from build123d import *

# Parameters (mm, degrees)
BOSS_EXTRUDE1_DEPTH = 5
SKETCH1_3_R         = 10
BOSS_EXTRUDE2_DEPTH = 2.5


with BuildPart() as part:
    # Sketch1 → Boss-Extrude1 (new, symmetric)
    with BuildSketch(Plane.XY):
        with BuildLine():
            Line((33, 85), (-32, 85))
            ThreePointArc((-32, 85), (-48.980483062, 75.567080721), (-49.943413521, 56.166319497))
            Line((-49.943413521, 56.166319497), (-17.943413521, -8.833680503))
            ThreePointArc((-17.943413521, -8.833680503), (0, -20), (17.943413521, -8.833680503))
            Line((17.943413521, -8.833680503), (50.833146609, 55.945780983))
            ThreePointArc((50.833146609, 55.945780983), (50.045298184, 75.46220865), (33, 85))
        make_face()
        with BuildLine():
            ThreePointArc((13.317368267, 6.90273152), (0, -15), (-13.317368267, 6.90273152))
            ThreePointArc((-13.317368267, 6.90273152), (-13.036984521, 33.958715313), (-34.650701601, 50.236064853))
            ThreePointArc((-34.650701601, 50.236064853), (-45.218522192, 72.090181314), (-21.166666667, 75.374916332))
            ThreePointArc((-21.166666667, 75.374916332), (0.5, 66.124748995), (22.166666667, 75.374916332))
            ThreePointArc((22.166666667, 75.374916332), (46.692872743, 71.124151864), (33.511719921, 50.008731117))
            ThreePointArc((33.511719921, 50.008731117), (12.785531325, 33.43522428), (13.317368267, 6.90273152))
        make_face(mode=Mode.SUBTRACT)
    extrude(amount=BOSS_EXTRUDE1_DEPTH, both=True)

    # Sketch1_3 → Boss-Extrude2 (add, symmetric)
    with BuildSketch(Plane.XY):
        with BuildLine():
            Line((-32, 85), (33, 85))
            ThreePointArc((33, 85), (50.045298184, 75.46220865), (50.833146609, 55.945780983))
            Line((50.833146609, 55.945780983), (17.943413521, -8.833680503))
            ThreePointArc((17.943413521, -8.833680503), (0, -20), (-17.943413521, -8.833680503))
            Line((-17.943413521, -8.833680503), (-49.943413521, 56.166319497))
            ThreePointArc((-49.943413521, 56.166319497), (-48.980483062, 75.567080721), (-32, 85))
        make_face()
        with Locations((-32, 65)):
            Circle(SKETCH1_3_R, mode=Mode.SUBTRACT)
        with Locations((33, 65)):
            Circle(SKETCH1_3_R, mode=Mode.SUBTRACT)
        Circle(SKETCH1_3_R, mode=Mode.SUBTRACT)
    extrude(amount=BOSS_EXTRUDE2_DEPTH, both=True)


solid = part.part
Check sheet for the modelled part. Datum: model origin and axes. Units: mm. A direction names the side the tool comes from. Round coordinates to 2 decimals unless told otherwise and drop trailing zeros. Write each loop counter-clockwise with the first axis right and the second up, starting at its lowest first coordinate (ties: lowest second). Pieces come first, ordered by that corner, then holes. Notation, with made-up numbers: (60, 78.25) -> (93, 78.25) arc R16 ccw to (93, 104.25) -> close; hole circle Ø11 at (72, -33). An arc over 180 degrees is marked (long way). Answer as CSV lines item,"result". Start each with the question number.
1) Material ranges on line 1 (Z direction, x = -9.5, y = 43); line 2 (Y direction, x = 0, z = 3.3); line 3 (Y direction, x = -32, z = -3.3), recorded low to high. Write a range as from..to.
2) Tool access check on faces 5 (the cylindrical face through (0, -15, 4)), 6 (the flat face through (-15, 37, -5)), 7 (the cylindrical face through (-12.87, 33.61, -3.73)). Record the directions out of +Z, -Z, +X, -X, +Y, -Y that give a thin tool (end or side, any length) a straight path to the whole face; none if there is none.
3) Section check B-B on y = 0. Enter the section's corners in (x, z).
4) Go/stop test with flat-tipped pins: P1, Ø24, axis at x = 0, y = 0, coming from the +Z side; P2, Ø1.5, axis at x = 34, z = -4, coming from the -Y side; P3, Ø1.5, axis at x = -22, z = 0.5, coming from the -Y side. Record where each tip stops, or that it passes through.
5) Release check for a two-part mould opening along Y. For faces 1 (the flat face through (-33.72, 23.21, 0.07)), 2 (the flat face through (1, 44, 2.5)), 3 (the cylindrical face through (-2.17, -9.76, -0.04)), 4 (the flat face through (0, 85, 0)) record: pulls with the +Y half, pulls with the -Y half, needs draft (parallel to the pull), parting line crosses it, or undercut.
6) Section check A-A on x = -37.5. Enter the section's corners in (y, z), and give its area (3 significant figures).
7) Section check C-C on y = 62.5. Enter the section's corners in (x, z).
8) Section check D-D on z = -3.75. Enter the section's corners in (x, y), and give its area (3 significant figures).
Found:
1,line 1,"z = -2.5..2.5"
1,line 2,"y = -20..-15, 66.13..85"
1,line 3,"y = 19.72..49.64, 80..85"
2,face 5,"+Z"
2,face 6,"-Z, +X, -X, +Y, -Y"
2,face 7,"-Z"
3,outline,"(-22.29, -5) -> (-15, -5) -> (-15, -2.5) -> (-10, -2.5) -> (-10, 2.5) -> (-15, 2.5) -> (-15, 5) -> (-22.29, 5) -> close; (10, -2.5) -> (15, -2.5) -> (15, -5) -> (22.43, -5) -> (22.43, 5) -> (15, 5) -> (15, 2.5) -> (10, 2.5) -> close"
4,P1,"stops at z = 2.5"
4,P2,"stops at y = 21.31"
4,P3,"stops at y = -2.12"
5,face 1,"pulls with the -Y half"
5,face 2,"undercut"
5,face 3,"undercut"
5,face 4,"pulls with the +Y half"
6,outline,"(30.89, -5) -> (51.04, -5) -> (51.04, -2.5) -> (56.65, -2.5) -> (56.65, 2.5) -> (51.04, 2.5) -> (51.04, 5) -> (30.89, 5) -> close; (73.35, -2.5) -> (78.96, -2.5) -> (78.96, -5) -> (84.23, -5) -> (84.23, 5) -> (78.96, 5) -> (78.96, 2.5) -> (73.35, 2.5) -> close"
6,area,"310 mm^2"
7,outline,"(-51.84, -5) -> (-46.79, -5) -> (-46.79, -2.5) -> (-41.68, -2.5) -> (-41.68, 2.5) -> (-46.79, 2.5) -> (-46.79, 5) -> (-51.84, 5) -> close; (-22.32, -2.5) -> (23.32, -2.5) -> (23.32, 2.5) -> (-22.32, 2.5) -> close; (42.68, -2.5) -> (47.79, -2.5) -> (47.79, -5) -> (52.84, -5) -> (52.84, 5) -> (47.79, 5) -> (47.79, 2.5) -> (42.68, 2.5) -> close"
8,outline,"(-49.94, 56.17) -> (-17.94, -8.83) arc R20 ccw to (17.94, -8.83) -> (50.83, 55.95) arc R20 ccw to (33, 85) -> (-32, 85) arc R20 ccw to start; hole (-34.65, 50.24) arc R30 cw to (-13.32, 6.9) arc R15 ccw (long way) to (13.32, 6.9) arc R30 cw to (33.51, 50.01) arc R15 ccw (long way) to (22.17, 75.37) arc R30 cw to (-21.17, 75.37) arc R15 ccw (long way) to start"
8,area,"3,640 mm^2"
